Answer from the drawing. Dimensions are ordinates in mm from the lowest x, y and z of the part. A direction names the side the tool comes from. Coordinates: 2 decimals unless noted, no trailing zeros. Write each loop counter-clockwise with the first axis right and the second up, starting at its lowest first coordinate (ties: lowest second). Pieces come first, ordered by that corner, then holes.
(1) Given pin 1 (1.5 mm diameter, centred on x = 4, z = 0.5, fed in from -Y) (1 decimal); pin 2 (6 mm diameter, centred on x = 8, y = 10.5, fed in from -Z), each flat-ended and moving along its own axis, determine where each tip first touches the part or whether it passes through.
(2) The part is cut by section C-C, the plane z = 1.3. State how many separate pieces and enclosed holes the cut face has.
(3) Straight lines are drawn through the part: line 1 along Z through (x, y) = (6, 16); line 2 along Y through (x, z) = (4.5, 1.9); line 3 along Y through (x, z) = (10.5, 2.8) (1 decimal). For each, find the intervals that lie inside material, in ascending order.
(4) Determine the mould class of the marked faces 1, 2 and 3 for opening direction X: pulls with the +X half, pulls with the -X half, needs draft (parallel to the pull), parting line crosses it, or undercut.
(5) The part is cut by section A-A, the plane y = 8. Determine the outline of the cut face in (x, z) (1 decimal).
(6) The part is cut by section B-B, the plane x = 10. Determine the outline of the cut face in (y, z).
(7) Which of the six approach directions +Z, -Z, +X, -X, +Y, -Y give full straight-line access (tool end or side, diameter ignored) to the marked faces 4 and 5?
(8) The part is cut by section D-D, the plane x = 17.25. Determine the outline of the cut face in (y, z).
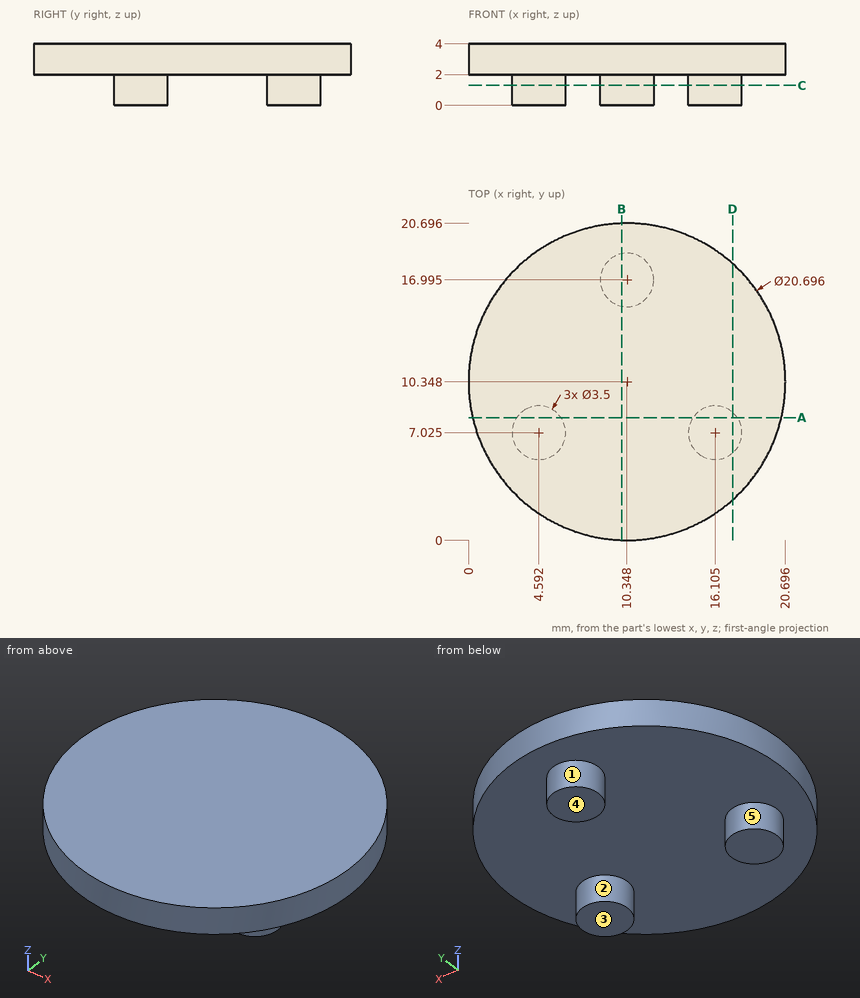
Computed:
1. pin 1: stops at y = 5.3
1. pin 2: stops at z = 2
2. separate pieces: 3
2. enclosed holes: 0
3. line 1: z = 2 to 4
3. line 2: y = 5.28 to 8.77
3. line 3: y = 0 to 20.7
4. face 1: parting line crosses it
4. face 2: undercut
4. face 3: needs draft
5. outline: (0.3, 2) - (3.1, 2) - (3.1, 0) - (6, 0) - (6, 2) - (14.7, 2) - (14.7, 0) - (17.6, 0) - (17.6, 2) - (20.4, 2) - (20.4, 4) - (0.3, 4) - close
6. outline: (0.01, 2) - (15.28, 2) - (15.28, 0) - (18.71, 0) - (18.71, 2) - (20.69, 2) - (20.69, 4) - (0.01, 4) - close
7. face 4: -Z, +X, -X, +Y, -Y
7. face 5: -Z
8. outline: (2.64, 2) - (5.7, 2) - (5.7, 0) - (8.35, 0) - (8.35, 2) - (18.06, 2) - (18.06, 4) - (2.64, 4) - close
